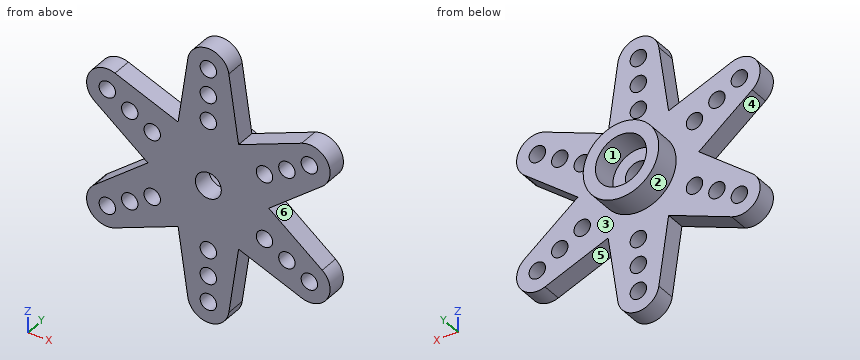
```python
from build123d import *

# Parameters (mm, degrees)
CROQUIS1_R              = 0.95
CROQUIS1_R_2            = 1.5
SALIENTE_EXTRUIR1_DEPTH = 2.3
CROQUIS2_R              = 4.375
CROQUIS2_R_2            = 2.95
SALIENTE_EXTRUIR2_DEPTH = 3


with BuildPart() as part:
    # Croquis1 → Saliente-Extruir1 (new body)
    with BuildSketch(Plane(origin=(0, 0, 0), x_dir=(1, 0, 0), z_dir=(0, 1, 0))):
        with BuildLine():
            Line((-3.5, 6.062177826), (-2.375316078, 13.843327148))
            ThreePointArc((-2.375316078, 13.843327148), (0, 15.9), (2.375316078, 13.843327148))
            Line((2.375316078, 13.843327148), (3.5, 6.062177826))
            Line((3.5, 6.062177826), (10.801014944, 8.978747639))
            ThreePointArc((10.801014944, 8.978747639), (13.76980392, 7.95), (13.176331022, 4.864579508))
            Line((13.176331022, 4.864579508), (7, 0))
            Line((7, 0), (13.176331022, -4.864579508))
            ThreePointArc((13.176331022, -4.864579508), (13.76980392, -7.95), (10.801014944, -8.978747639))
            Line((10.801014944, -8.978747639), (3.5, -6.062177826))
            Line((3.5, -6.062177826), (2.375316078, -13.843327148))
            ThreePointArc((2.375316078, -13.843327148), (0, -15.9), (-2.375316078, -13.843327148))
            Line((-2.375316078, -13.843327148), (-3.5, -6.062177826))
            Line((-3.5, -6.062177826), (-10.801014944, -8.978747639))
            ThreePointArc((-10.801014944, -8.978747639), (-13.76980392, -7.95), (-13.176331022, -4.864579508))
            Line((-13.176331022, -4.864579508), (-7, 0))
            Line((-7, 0), (-13.176331022, 4.864579508))
            ThreePointArc((-13.176331022, 4.864579508), (-13.76980392, 7.95), (-10.801014944, 8.978747639))
            Line((-10.801014944, 8.978747639), (-3.5, 6.062177826))
        make_face()
        with Locations(Location((0, 13.5, 0), (0, 0, 270))):
            Circle(CROQUIS1_R, mode=Mode.SUBTRACT)
        with Locations(Location((0, 10.5, 0), (0, 0, 270))):
            Circle(CROQUIS1_R, mode=Mode.SUBTRACT)
        with Locations(Location((0, 7.5, 0), (0, 0, 270))):
            Circle(CROQUIS1_R, mode=Mode.SUBTRACT)
        with Locations(Location((11.691342951, 6.75, 0), (0, 0, 270))):
            Circle(CROQUIS1_R, mode=Mode.SUBTRACT)
        with Locations(Location((9.09326674, 5.25, 0), (0, 0, 270))):
            Circle(CROQUIS1_R, mode=Mode.SUBTRACT)
        with Locations(Location((6.495190528, 3.75, 0), (0, 0, 270))):
            Circle(CROQUIS1_R, mode=Mode.SUBTRACT)
        with Locations(Location((11.691342951, -6.75, 0), (0, 0, 270))):
            Circle(CROQUIS1_R, mode=Mode.SUBTRACT)
        with Locations(Location((9.09326674, -5.25, 0), (0, 0, 270))):
            Circle(CROQUIS1_R, mode=Mode.SUBTRACT)
        with Locations(Location((6.495190528, -3.75, 0), (0, 0, 270))):
            Circle(CROQUIS1_R, mode=Mode.SUBTRACT)
        with Locations(Location((0, -13.5, 0), (0, 0, 270))):
            Circle(CROQUIS1_R, mode=Mode.SUBTRACT)
        with Locations(Location((0, -10.5, 0), (0, 0, 270))):
            Circle(CROQUIS1_R, mode=Mode.SUBTRACT)
        with Locations(Location((0, -7.5, 0), (0, 0, 270))):
            Circle(CROQUIS1_R, mode=Mode.SUBTRACT)
        with Locations(Location((-11.691342951, -6.75, 0), (0, 0, 270))):
            Circle(CROQUIS1_R, mode=Mode.SUBTRACT)
        with Locations(Location((-9.09326674, -5.25, 0), (0, 0, 270))):
            Circle(CROQUIS1_R, mode=Mode.SUBTRACT)
        with Locations(Location((-6.495190528, -3.75, 0), (0, 0, 270))):
            Circle(CROQUIS1_R, mode=Mode.SUBTRACT)
        with Locations(Location((-11.691342951, 6.75, 0), (0, 0, 270))):
            Circle(CROQUIS1_R, mode=Mode.SUBTRACT)
        with Locations(Location((-9.09326674, 5.25, 0), (0, 0, 270))):
            Circle(CROQUIS1_R, mode=Mode.SUBTRACT)
        with Locations(Location((-6.495190528, 3.75, 0), (0, 0, 270))):
            Circle(CROQUIS1_R, mode=Mode.SUBTRACT)
        with Locations(Location((0, 0, 0), (0, 0, 270))):
            Circle(CROQUIS1_R_2, mode=Mode.SUBTRACT)
    extrude(amount=SALIENTE_EXTRUIR1_DEPTH)

    # Croquis2 → Saliente-Extruir2 (add)
    with BuildSketch(Plane(origin=(0, 2.3, 0), x_dir=(1, 0, 0), z_dir=(0, 1, 0))):
        with Locations(Location((0, 0, 0), (0, 0, 270))):
            Circle(CROQUIS2_R)
        with Locations(Location((0, 0, 0), (0, 0, 270))):
            Circle(CROQUIS2_R_2, mode=Mode.SUBTRACT)
    extrude(amount=SALIENTE_EXTRUIR2_DEPTH)


solid = part.part
```
Verification items for the finished model (mm, model axes). Face numbers are marked on the shaded views. A direction names the side the tool comes from. Coordinates: 2 decimals unless noted, no trailing zeros. Loops run counter-clockwise (first coordinate to the right, second up) from the corner with the lowest first, then second, coordinate; pieces in that order, holes last. Notation, with made-up numbers: (33, 1.5) - (82, 1.5) arc R21 cw to (82, 38.5) - close; hole circle Ø9 at (24.25, 24.5). An arc over 180 degrees is marked (long way). Put each result on its own line as item: value.
Item 1: Scan lines: line 1 along X through (y, z) = (1.2, -5.25); line 2 along Y through (x, z) = (4.75, -1); line 3 along X through (y, z) = (0.95, -3.5). Record each from-to range of solid material in increasing order.
Conclusion:
line 1: x = -13.56 to -10.04, -8.14 to 8.14, 10.04 to 13.56
line 2: y = 0 to 2.3
line 3: x = -11.44 to -7.41, -5.58 to 5.58, 7.41 to 11.44
Item 2: Section check C-C (x = 0). Give the number of separate pieces and of enclosed holes in the cut face, then the cut area to 3 significant figures.
Conclusion:
separate pieces: 8
enclosed holes: 0
area: 48.6 mm2
Item 3: Draft check along X on the marked faces 1, 2 and 3. Enter one of: pulls with the +X half, pulls with the -X half, needs draft (parallel to the pull), parting line crosses it, or undercut.
Conclusion:
face 1: undercut
face 2: parting line crosses it
face 3: needs draft
Item 4: Set-up check for the marked faces 4, 5 and 6: record each of +Z, -Z, +X, -X, +Y, -Y from which the full face is reachable in a straight line by a thin tool's end or side.
Conclusion:
face 4: -X, +Y, -Y
face 5: -Z, +Y, -Y
face 6: +X, +Y, -Y
Item 5: Section check B-B (z = -5.25). Enter the section's corners in (x, y).
Conclusion:
outline: (-13.56, 0) - (-10.04, 0) - (-10.04, 2.3) - (-13.56, 2.3) - close; (-8.14, 0) - (8.14, 0) - (8.14, 2.3) - (-8.14, 2.3) - close; (10.04, 0) - (13.56, 0) - (13.56, 2.3) - (10.04, 2.3) - close
Item 6: Section check D-D (y = 4.1). Enter the section's corners in (x, z) (3 decimals).
Conclusion:
outline: circle Ø8.75 at (0, 0); hole circle Ø5.9 at (0, 0)
Item 7: Gauge pin test, flat ends, axial feed: pin 1 Ø3 at (x, y) = (-2, 1) entering from +Z; pin 2 Ø2.5 at (x, z) = (-6.5, 3.75) entering from +Y. Record the tip position at first contact, or that the pin passes through.
Conclusion:
pin 1: stops at z = 15.85
pin 2: stops at y = 2.3
Item 8: Section check A-A (z = -11). Enter the section's corners in (x, y).
Conclusion:
outline: (-2.79, 0) - (-0.81, 0) - (-0.81, 2.3) - (-2.79, 2.3) - close; (0.81, 0) - (2.79, 0) - (2.79, 2.3) - (0.81, 2.3) - close
